The drawing under review shows one solid part. Ordinate dimensions are in mm from its lowest x, y, z. A direction names the side the tool comes from. Give positions to 0.01 mm unless a question says otherwise; leave off trailing zeros. Loops run counter-clockwise (first coordinate to the right, second up) from the corner with the lowest first, then second, coordinate; pieces in that order, holes last. Notation, with made-up numbers: M 5,10 L 61,10 A38 cw 61,48 Z; hole C -28.75,35 d1. An arc over 180 degrees is marked long. Put each result on its own line as item: value. Start each with the question number.
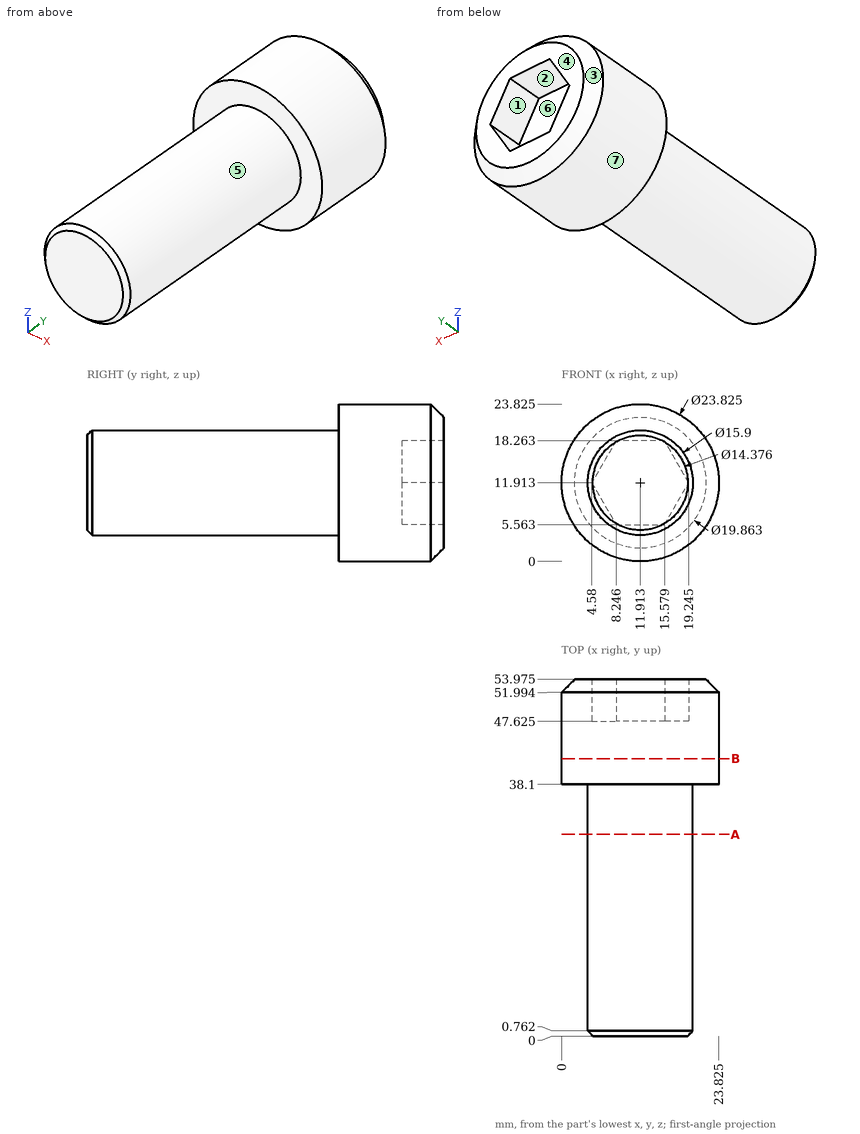
(1) For the marked faces 5, 6 and 7, list the 3-axis set-ups (+Z, -Z, +X, -X, +Y, -Y) from which the entire face can be reached by the end or side of a thin tool; tool diameter is ignored.
(2) We need section A-A, the plane y = 30.5. Write out the cut boundary in (x, z).
(3) We need section B-B, the plane y = 42. Write out the cut boundary in (x, z) (1 decimal).
(4) To check wall thickness, follow L1, parallel to Y at x = 5.75, z = 4.25 (1 decimal); L2, parallel to Y at x = 6.75, z = 9.75 (1 decimal); L3, parallel to Z at x = 17.5, y = 50.5 (1 decimal). State the ranges of each line that lie inside material, in increasing order. Write a range as [from, to].
(5) Insertion check: pin 1 (5 mm diameter, centred on y = 8.5, z = 10.5, fed in from +X); pin 2 (3 mm diameter, centred on x = 9, y = 42, fed in from +Z); pin 3 (2 mm diameter, centred on x = 2.5, z = 3, fed in from -Y); pin 4 (5 mm diameter, centred on y = 42, z = 15.5, fed in from -X). Each pin has a flat end and moves straight along its axis. Give the tip position at first contact, or say it passes through.
(6) Draft analysis for pull direction Z (two halves, no side actions). For the marked faces 1, 2, 3 and 4, state which applies: +Z half, -Z half, draft (parallel to the pull), parting line (faces both ways), or undercut.
Check sheet entries:
1. face 5: -Y
1. face 6: +Y
1. face 7: +Y, -Y
2. outline: C 11.91,11.91 d15.9
3. outline: C 11.9,11.9 d23.8
4. L1: y = [38.1, 54]
4. L2: y = [0, 47.6]
4. L3: z = [1.4, 8.9], [14.9, 22.4]
5. pin 1: stops at x = 19.86
5. pin 2: stops at z = 23.74
5. pin 3: passes through
5. pin 4: stops at x = 0.05
6. face 1: undercut
6. face 2: undercut
6. face 3: parting line
6. face 4: draft
